```python
from build123d import *

# Parameters (mm, degrees)
SKETCH1_R           = 1.6
BOSS_EXTRUDE1_DEPTH = 3
SKETCH2_W           = 10
SKETCH2_H           = 10
BOSS_EXTRUDE2_DEPTH = 42
CHAMFER1_SIZE       = 5
SKETCH3_R           = 2.1
CUT_EXTRUDE1_DEPTH  = 52
SKETCH4_R           = 2.65
CUT_EXTRUDE2_DEPTH  = 0.5


with BuildPart() as part:
    # Sketch1 → Boss-Extrude1 (new body)
    with BuildSketch(Plane(origin=(0, 0, 0), x_dir=(1, 0, 0), z_dir=(0, 1, 0))):
        Polygon((-6.512396694, 9.685950413), (1.487603306, 9.685950413), (26.487603306, 9.685950413), (26.487603306, -40.314049587), (1.487603306, -40.314049587), (-6.512396694, -40.314049587), align=None)
        with Locations(Location((-1.962396694, -35.764049587, 0), (0, 0, 270))):
            Circle(SKETCH1_R, mode=Mode.SUBTRACT)
        with Locations(Location((-1.962396694, 5.135950413, 0), (0, 0, 270))):
            Circle(SKETCH1_R, mode=Mode.SUBTRACT)
    extrude(amount=BOSS_EXTRUDE1_DEPTH)

    # Sketch2 → Boss-Extrude2 (add)
    with BuildSketch(Plane(origin=(0, 3, 0), x_dir=(1, 0, 0), z_dir=(0, 1, 0))):
        with Locations((21.487603306, -35.314049587)):
            Rectangle(SKETCH2_W, SKETCH2_H)
        with Locations((21.487603306, 4.685950413)):
            Rectangle(SKETCH2_W, SKETCH2_H)
    extrude(amount=BOSS_EXTRUDE2_DEPTH)

    # Chamfer1
    chamfer1_edges = [part.edges().sort_by_distance(p)[0] for p in [
        (21.487603306, 3, 30.314049587),
        (16.487603306, 3, 35.314049587),
        (16.487603306, 3, -4.685950413),
        (21.487603306, 3, 0.314049587),
    ]]
    chamfer(chamfer1_edges, length=CHAMFER1_SIZE)

    # Sketch3 → Cut-Extrude1 (cut)
    with BuildSketch(Plane(origin=(0, 45, 0), x_dir=(1, 0, 0), z_dir=(0, 1, 0))):
        with Locations(Location((22.537603306, -36.364049587, 0), (0, 0, 270))):
            Circle(SKETCH3_R)
        with Locations(Location((22.537603306, 5.735950413, 0), (0, 0, 270))):
            Circle(SKETCH3_R)
    extrude(amount=-CUT_EXTRUDE1_DEPTH, mode=Mode.SUBTRACT)

    # Sketch4 → Cut-Extrude2 (cut)
    with BuildSketch(Plane(origin=(0, 45, 0), x_dir=(1, 0, 0), z_dir=(0, 1, 0))):
        with Locations(Location((22.537603306, -36.364049587, 0), (0, 0, 270))):
            Circle(SKETCH4_R)
        with Locations(Location((22.537603306, 5.735950413, 0), (0, 0, 270))):
            Circle(SKETCH4_R)
    cut_extrude2 = extrude(amount=-CUT_EXTRUDE2_DEPTH, mode=Mode.SUBTRACT)

    # Mirror1: Cut-Extrude2 across plane
    add(cut_extrude2.mirror(Plane(origin=(0, 22.5, 0), x_dir=(0, 0, 1), z_dir=(0, -1, 0))), mode=Mode.SUBTRACT)


solid = part.part
```
Geometry: final body of the model. Coordinates: model frame, mm. A direction names the side the tool comes from. Coordinates: 2 decimals unless noted, no trailing zeros. Order: outer loops, then holes, each group sorted by start corner. A loop starts at its lowest first (then second) coordinate and runs counter-clockwise, first axis right, second up. Notation, with made-up numbers: M 70.5,71.5 L 91.5,71.5 A18 cw 91.5,97.5 Z; hole C 43,81 d9. An arc over 180 degrees is marked long. Answer in a Markdown table with one row per item. Add a question column.
Q1. Section query D-D on z = 12. Return the cut outline in (x, y), and give its area (3 significant figures).
Q2. Mould query, pull axis X, two halves, no side actions, for faces 1 (the flat face through (26.488, 22, -1)), 2 (the cylindrical face through (-2.58, 1.48, -3.66)), 3 (the flat face through (10, 0, 15)). Classes: released by +X, released by -X, zero draft, split by the parting line, or undercut.
Q3. Line query: L1, parallel to Z at x = 19, y = 15; L2, parallel to Z at x = 23.5, y = 36.5; L3, parallel to Z at x = 21, y = 3.5. Output: solid intervals per line, ascending.
Q4. Reachability of faces 4 (the flat face through (21, 0.5, -4)), 5 (the flat face through (20.549, 5.465, 2.849)), 6 (the cylindrical face through (22.654, 44.754, 33.717)) from +Z, -Z, +X, -X, +Y, -Y: full face, straight path, thin tool, end or side. Return the list, or none.
Q5. Contact query for flat-ended pins moving along their axis: P1, Ø1, axis at x = 7.5, z = 17.5, coming from the -Y side; P2, Ø8, axis at y = 19, z = -7, coming from the -X side; P3, Ø10, axis at x = 8.5, z = 3.5, coming from the +Y side; P4, Ø4, axis at x = -1.96, z = -5.14, coming from the +Y side. Output: stop coordinate, or through.
Q6. Section query A-A on y = 24. Return the cut outline in (x, z).
Q7. Section query B-B on z = 32.5. Return the cut outline in (x, y).
Q8. Section query C-C on x = 7. Return the cut outline in (y, z), and give its area (3 significant figures).
Completed:
| question | item | result |
|---|---|---|
| 1 | outline | M -6.51,0 L 26.49,0 L 26.49,3 L -6.51,3 Z |
| 1 | area | 99.0 mm2 |
| 2 | face 1 | released by +X |
| 2 | face 2 | undercut |
| 2 | face 3 | zero draft |
| 3 | L1 | z = -9.69 to 0.31, 30.31 to 40.31 |
| 3 | L2 | z = -9.69 to -7.6, -3.87 to 0.31, 30.31 to 34.5, 38.23 to 40.31 |
| 3 | L3 | z = -9.69 to -7.17, -4.31 to 4.81, 25.81 to 34.93, 37.79 to 40.31 |
| 4 | face 4 | -Y |
| 4 | face 5 | +X, -X, +Y |
| 4 | face 6 | +Y |
| 5 | P1 | stops at y = 0 |
| 5 | P2 | stops at x = 16.49 |
| 5 | P3 | stops at y = 5.01 |
| 5 | P4 | stops at y = 3 |
| 6 | outline | M 16.49,-9.69 L 26.49,-9.69 L 26.49,0.31 L 16.49,0.31 Z; M 16.49,30.31 L 26.49,30.31 L 26.49,40.31 L 16.49,40.31 Z; hole C 22.54,-5.74 d4.2; hole C 22.54,36.36 d4.2 |
| 7 | outline | M -6.51,0 L 26.49,0 L 26.49,45 L 16.49,45 L 16.49,8 L 11.49,3 L -6.51,3 Z |
| 8 | outline | M 0,-9.69 L 3,-9.69 L 3,40.31 L 0,40.31 Z |
| 8 | area | 150 mm2 |
